from build123d import *

# Parameters (mm, degrees)
SKETCH_1_W          = 22
SKETCH_1_H          = 41
EXTRUDE_1_DEPTH     = 3
SKETCH_2_W          = 5
SKETCH_2_H          = 4
EXTRUDE_2_DEPTH     = 3
SKETCH_3_W          = 6
SKETCH_3_H          = 10
CUT_EXTRUDE_1_DEPTH = 10
SKETCH_4_R          = 1.5
CUT_EXTRUDE_2_DEPTH = 10
SKETCH_5_R          = 11
CUT_EXTRUDE_3_DEPTH = 10
FILLET_1_R          = 2


with BuildPart() as part:
    # 草图1 → 凸台-拉伸1 (new body)
    with BuildSketch(Plane(origin=(0, 0, 0), x_dir=(1, 0, 0), z_dir=(0, 1, 0))):
        Rectangle(SKETCH_1_W, SKETCH_1_H)
    extrude(amount=EXTRUDE_1_DEPTH)

    # 草图2 → 凸台-拉伸2 (add)
    with BuildSketch(Plane(origin=(0, 3, 0), x_dir=(1, 0, 0), z_dir=(0, 1, 0))):
        with Locations((-6.5, 22.5)):
            Rectangle(SKETCH_2_W, SKETCH_2_H)
        with Locations((6.5, 22.5)):
            Rectangle(SKETCH_2_W, SKETCH_2_H)
        with Locations((6.5, -22.5)):
            Rectangle(SKETCH_2_W, SKETCH_2_H)
        with Locations((-6.5, -22.5)):
            Rectangle(SKETCH_2_W, SKETCH_2_H)
    extrude(amount=-EXTRUDE_2_DEPTH)

    # 草图3 → 切除-拉伸1 (cut)
    with BuildSketch(Plane.XZ):
        with Locations((1.906204118, -9.5)):
            Rectangle(SKETCH_3_W, SKETCH_3_H)
    extrude(amount=-CUT_EXTRUDE_1_DEPTH, mode=Mode.SUBTRACT)

    # 草图4 → 切除-拉伸2 (cut)
    with BuildSketch(Plane.XZ):
        with Locations(Location((-6.5, 18, 0), (0, 0, 270))):
            Circle(SKETCH_4_R)
        with Locations(Location((8.5, 18, 0), (0, 0, 270))):
            Circle(SKETCH_4_R)
        with Locations(Location((-6.5, 3, 0), (0, 0, 270))):
            Circle(SKETCH_4_R)
        with Locations(Location((8.5, 3, 0), (0, 0, 270))):
            Circle(SKETCH_4_R)
    extrude(amount=-CUT_EXTRUDE_2_DEPTH, mode=Mode.SUBTRACT)

    # 草图5 → 切除-拉伸3 (cut)
    with BuildSketch(Plane.XZ):
        with Locations((-18.5, 10.5)):
            Circle(SKETCH_5_R)
    extrude(amount=-CUT_EXTRUDE_3_DEPTH, mode=Mode.SUBTRACT)

    # 圆角1
    fillet_1_edges = [part.edges().sort_by_distance(p)[0] for p in [
        (-11, 1.5, 18.54673847),
        (-11, 1.5, 2.45326153),
    ]]
    fillet(fillet_1_edges, radius=FILLET_1_R)


solid = part.part
Read the model definition and answer for the solid it produces. Units are mm, in the model's axes. A direction names the side the tool comes from. Give positions to 0.01 mm unless a question says otherwise; leave off trailing zeros. Loops run counter-clockwise (first coordinate to the right, second up) from the corner with the lowest first, then second, coordinate; pieces in that order, holes last. Notation, with made-up numbers: (-15.75, -9) -> (35.25, -9) arc R19 cw to (35.25, -3) -> close; hole circle Ø3 at (82.5, -34). An arc over 180 degrees is marked (long way). Answer as CSV lines item,"result".
Item 1: Find section D-D on z = 9.5. Give the vertices of the cut face in (x, y), plus the area to 3 significant figures.
Returned:
outline,"(-7.55, 0) -> (11, 0) -> (11, 3) -> (-7.55, 3) -> close"
area,"55.6 mm²"
Item 2: Find section A-A on x = 1.5. Give the vertices of the cut face in (y, z).
Returned:
outline,"(0, -20.5) -> (3, -20.5) -> (3, -14.5) -> (0, -14.5) -> close; (0, -4.5) -> (3, -4.5) -> (3, 20.5) -> (0, 20.5) -> close"
Item 3: Find section C-C on x = -6.5. Give the vertices of the cut face in (y, z).
Returned:
outline,"(0, -24.5) -> (3, -24.5) -> (3, 1.5) -> (0, 1.5) -> close; (0, 4.5) -> (3, 4.5) -> (3, 16.5) -> (0, 16.5) -> close; (0, 19.5) -> (3, 19.5) -> (3, 24.5) -> (0, 24.5) -> close"
Item 4: For faces 4 (the face through (9, 2, 23)), 5 (the face through (9, 2, -22)), 6 (the face through (2, 1, -4.5)), 7 (the face through (-10, 1, 20.5)), 8 (the face through (4, 2, 23)), determine the directions among +Z, -Z, +X, -X, +Y, -Y from which every point of the face is accessible in a straight line to the end or side of a thin tool.
Returned:
face 4,"+Z, +X, +Y, -Y"
face 5,"-Z, +X, +Y, -Y"
face 6,"+Y, -Y"
face 7,"+Z, -X, +Y, -Y"
face 8,"+Z, +Y, -Y"
Item 5: Each of these flat-tipped pins is pushed along its axis until it touches: pin 1 (1.5 mm diameter, centred on y = 1.5, z = -21.5, fed in from -X); pin 2 (1.5 mm diameter, centred on y = 1.5, z = -23, fed in from +X); pin 3 (1.5 mm diameter, centred on x = 2, y = 2, fed in from +Z). Where does it stop, or does it pass through?
Returned:
pin 1,"stops at x = -9"
pin 2,"stops at x = 9"
pin 3,"stops at z = 20.5"
Item 6: Consider line 1 (X direction, y = 1.95, z = 3); line 2 (X direction, y = 0.7, z = 4); line 3 (Z direction, x = 3.5, y = 0.2). Determine where each line is inside the solid, lowest interval first. Write a range as [from, to].
Returned:
line 1,"x = [-10.45, -8], [-5, 7], [10, 11]"
line 2,"x = [-9.63, -7.62], [-5.38, 7.38], [9.62, 11]"
line 3,"z = [-20.5, -14.5], [-4.5, 20.5]"
Item 7: Determine the mould class of faces 1 (the face through (0, 1, 20.5)), 2 (the face through (4, 2, -22)), 3 (the face through (-7.5, 1.5, 10.4)) for opening direction Z: +Z half, -Z half, draft (parallel to the pull), parting line (faces both ways), or undercut.
Returned:
face 1,"+Z half"
face 2,"draft"
face 3,"undercut"
Item 8: Find section B-B on y = 2.3. State how many separate pieces and enclosed holes the cut face has, plus the area to 3 significant figures.
Returned:
separate pieces,"1"
enclosed holes,"5"
area,"855 mm²"
